CAD build for the part. Positions are in the model's coordinates, mm. A direction names the side the tool comes from. Give positions to 0.01 mm unless a question says otherwise; leave off trailing zeros. Write each loop counter-clockwise with the first axis right and the second up, starting at its lowest first coordinate (ties: lowest second). Pieces come first, ordered by that corner, then holes. Notation, with made-up numbers: (49.25, 10.25) -> (103.25, 10.25) arc R11 ccw to (103.25, 28.25) -> close; hole circle Ø7 at (6.5, -8.75). An arc over 180 degrees is marked (long way). Answer as a JSON object with one key per item and string values.
```python
from build123d import *

# Parameters (mm, degrees)
BOSS_EXTRUDE1_DEPTH = 25.4
SKETCH2_W           = 27.340735927
SKETCH2_H           = 19.391580929
CUT_EXTRUDE1_DEPTH  = 50
SKETCH4_R           = 1.1938
CUT_EXTRUDE2_DEPTH  = 50


with BuildPart() as part:
    # Sketch1 → Boss-Extrude1 (new body)
    with BuildSketch(Plane.XY):
        with BuildLine():
            Line((-8.516561995, -2.000000064), (-8.748247165, -2.000000064))
            Line((-8.748247165, -2.000000064), (-8.748247165, 2))
            Line((-8.748247165, 2), (-8.51656201, 2))
            ThreePointArc((-8.51656201, 2), (0, 8.748247165), (8.51656201, 2))
            Line((8.51656201, 2), (8.748247165, 2))
            Line((8.748247165, 2), (8.748247165, -2.000000064))
            Line((8.748247165, -2.000000064), (8.516561995, -2.000000064))
            ThreePointArc((8.516561995, -2.000000064), (0, -8.748247165), (-8.516561995, -2.000000064))
        make_face()
        with BuildLine():
            Line((-5.088737122, 2), (-5.088737097, -2.000000064))
            ThreePointArc((-5.088737097, -2.000000064), (0, -5.467654478), (5.088737097, -2.000000064))
            Line((5.088737097, -2.000000064), (5.088737122, 2))
            ThreePointArc((5.088737122, 2), (0, 5.467654478), (-5.088737122, 2))
        make_face(mode=Mode.SUBTRACT)
    extrude(amount=-BOSS_EXTRUDE1_DEPTH)

    # Sketch2 → Cut-Extrude1 (cut)
    with BuildSketch(Plane.XY):
        with Locations((-11.729632037, -0.299788476)):
            Rectangle(SKETCH2_W, SKETCH2_H)
    extrude(amount=-CUT_EXTRUDE1_DEPTH, mode=Mode.SUBTRACT)

    # Sketch4 → Cut-Extrude2 (cut)
    with BuildSketch(Plane(origin=(11.288247165, 0, 0), x_dir=(0, 0, -1), z_dir=(1, 0, 0))):
        with Locations((4.4958, 0)):
            Circle(SKETCH4_R)
        with Locations((8.9662, 0)):
            Circle(SKETCH4_R)
    extrude(amount=-CUT_EXTRUDE2_DEPTH, mode=Mode.SUBTRACT)


solid = part.part
```
1) Slice it at B-B (y = 0). List the corners of the cut face in (x, z), then the cut area to 3 significant figures.
Model answer:
{"outline": "(5.09, -25.4) -> (8.75, -25.4) -> (8.75, -10.16) -> (5.09, -10.16) -> close; (5.09, -7.77) -> (8.75, -7.77) -> (8.75, -5.69) -> (5.09, -5.69) -> close; (5.09, -3.3) -> (8.75, -3.3) -> (8.75, 0) -> (5.09, 0) -> close", "area": "75.5 mm2"}
2) Slice it at D-D (z = -17.25). List the corners of the cut face in (x, y).
Model answer:
{"outline": "(1.94, -8.53) arc R8.75 ccw to (8.52, -2) -> (8.75, -2) -> (8.75, 2) -> (8.52, 2) arc R8.75 ccw to (1.94, 8.53) -> (1.94, 5.11) arc R5.47 cw to (5.09, 2) -> (5.09, -2) arc R5.47 cw to (1.94, -5.11) -> close"}
3) Wall check: probe 1 along X at (y, z) = (-0.5, -23.25); probe 2 along Z at (x, y) = (7.75, 0.75) (3 decimals); probe 3 along Y at (x, z) = (6.75, -8.5) (3 decimals). Give the ranges that are in metal, low to high.
Model answer:
{"probe 1": "x = 5.09 to 8.75", "probe 2": "z = -25.4 to -9.895, -8.037 to -5.425, -3.567 to 0", "probe 3": "y = -5.565 to -1.099, 1.099 to 5.565"}
4) Pin check, flat tips, straight feed: pin 1 (1 mm diameter, centred on x = 3.5, z = -21, fed in from -Y); pin 2 (2 mm diameter, centred on y = 0, z = -15, fed in from -X); pin 3 (3 mm diameter, centred on y = 1, z = -15.5, fed in from -X). Stop position of each tip, or through.
Model answer:
{"pin 1": "stops at y = -8.22", "pin 2": "stops at x = 5.09", "pin 3": "stops at x = 4.86"}
5) Slice it at A-A (x = 4.75). List the corners of the cut face in (y, z).
Model answer:
{"outline": "(-7.35, -25.4) -> (-2.71, -25.4) -> (-2.71, 0) -> (-7.35, 0) -> close; (2.71, -25.4) -> (7.35, -25.4) -> (7.35, 0) -> (2.71, 0) -> close"}
6) Mould opens along Z. For faces 3 (the cylindrical face through (6.944, 0.052, -3.303)), 4 (the cylindrical face through (6.944, 0.052, -7.774)), 5 (the flat face through (1.941, 7, -13)), 6 (the flat face through (5.4, 0.1, 0)) say: released by +Z, released by -Z, zero draft, split by the parting line, or undercut.
Model answer:
{"face 3": "undercut", "face 4": "undercut", "face 5": "zero draft", "face 6": "released by +Z"}
7) 3-axis set-ups, long thin cutter, end or side, ignore diameter. For faces 1 (the cylindrical face through (6.116, 6.255, -12.522)), 2 (the flat face through (5.089, 0, -13)): which of +Z, -Z, +X, -X, +Y, -Y reach the whole face in a straight line?
Model answer:
{"face 1": "+Z, -Z, +X, +Y", "face 2": "+Z, -Z, -X"}
8) Slice it at C-C (z = -3.75). List the corners of the cut face in (x, y), then the cut area to 3 significant figures.
Model answer:
{"outline": "(1.94, -8.53) arc R8.75 ccw to (8.52, -2) -> (8.75, -2) -> (8.75, -0.93) -> (5.09, -0.93) -> (5.09, -2) arc R5.47 cw to (1.94, -5.11) -> close; (1.94, 5.11) arc R5.47 cw to (5.09, 2) -> (5.09, 0.93) -> (8.75, 0.93) -> (8.75, 2) -> (8.52, 2) arc R8.75 ccw to (1.94, 8.53) -> close", "area": "54.9 mm2"}
